from build123d import *

# Parameters (mm, degrees)
F1_DEPTH = 11.5
F2_R     = 4.5
F3_DEPTH = 11.501
F4_R     = 3
F5_DEPTH = 10


with BuildPart() as f1:
    # F0 (on Front) → F1 (new body)
    with BuildSketch(Plane.XZ):
        Polygon((-44.5, 15.5), (-41.5, 0), (41.5, 0), (44.5, 15.5), align=None)
    extrude(amount=F1_DEPTH)

    # F2 (on face) → F3 (cut, through all)
    with BuildSketch(Plane(origin=(0, 0, 0), x_dir=(-1, 0, 0), z_dir=(0, 1, 0))):
        with Locations((0, 7.5)):
            Circle(F2_R)
    extrude(amount=-F3_DEPTH, mode=Mode.SUBTRACT)

    # F4 (on face) → F5 (cut)
    with BuildSketch(Plane(origin=(0, 0, 0), x_dir=(1, 0, 0), z_dir=(0, 0, -1))):
        with Locations((0, 5.75)):
            Circle(F4_R)
    extrude(amount=-F5_DEPTH, mode=Mode.SUBTRACT)


solid = f1.part
The listing builds one solid part. Answer for the finished solid, in the listing's coordinates (mm). Round coordinates to 2 decimals unless told otherwise and drop trailing zeros. Write each loop counter-clockwise with the first axis right and the second up, starting at its lowest first coordinate (ties: lowest second). Pieces come first, ordered by that corner, then holes. Notation, with made-up numbers: M 3,62 L 48,62 A29 ccw 48,89 Z; hole C 13.25,48.25 d3. An arc over 180 degrees is marked long. Write each question's results on one line, items separated by ' | '. Start each with the question number.
(1) The part is cut by section B-B, the plane y = -1.5. Write down the section's boundary in (x, z), and give its area (3 significant figures).
(2) The part is cut by section C-C, the plane z = 10.5. Write down the section's boundary in (x, y).
(3) The part is cut by section D-D, the plane y = -5.75. Write down the section's boundary in (x, z), and give its area (3 significant figures).
(4) Find the intervals of material crossed by line 1 (Z direction, x = 0, y = -8.5); line 2 (X direction, y = -6.5, z = 10.5); line 3 (Z direction, x = -1, y = -9.5), in increasing order.
(5) The part is cut by section A-A, the plane x = 0. Write down the section's boundary in (y, z).
(6) Determine the mould class of faces 1 (the flat face through (-0.6, 0, 2.7)), 2 (the flat face through (42.98, -5.67, 7.64)), 3 (the cylindrical face through (2.77, -4.6, 1.58)), 4 (the flat face through (-0.6, -11.5, 2.7)) for opening direction Y: +Y half, -Y half, draft (parallel to the pull), parting line (faces both ways), or undercut.
(7) Each of these flat-tipped pins is pushed along its axis until it touches: P1, Ø2, axis at x = 19.5, z = 11, coming from the +Y side; P2, Ø1.5, axis at y = -4, z = 5, coming from the +X side; P3, Ø1, axis at y = -2, z = 7, coming from the -X side. Where does it stop, or does it pass through?
Worked answers:
1) outline: M -44.5,15.5 L -41.5,0 L 41.5,0 L 44.5,15.5 Z; hole C 0,7.5 d9 | area: 1,270 mm²
2) outline: M -43.53,-11.5 L -3.35,-11.5 L -3.35,0 L -43.53,0 Z; M 3.35,-11.5 L 43.53,-11.5 L 43.53,0 L 3.35,0 Z
3) outline: M -44.5,15.5 L -41.5,0 L -3,0 L -3,4.15 A4.5 cw long 3,4.15 L 3,0 L 41.5,0 L 44.5,15.5 Z | area: 1,250 mm²
4) line 1: z = 12 to 15.5 | line 2: x = -43.53 to -3.35, 3.35 to 43.53 | line 3: z = 0 to 3.11, 11.89 to 15.5
5) outline: M -11.5,0 L -8.75,0 L -8.75,3 L -11.5,3 Z; M -11.5,12 L 0,12 L 0,15.5 L -11.5,15.5 Z; M -2.75,0 L 0,0 L 0,3 L -2.75,3 Z
6) face 1: +Y half | face 2: draft | face 3: undercut | face 4: -Y half
7) P1: stops at y = 0 | P2: stops at x = 42.61 | P3: stops at x = -42.95
